The model under review builds one solid part; all positions refer to its coordinate system, in mm. A direction names the side the tool comes from. Give positions to 0.01 mm unless a question says otherwise; leave off trailing zeros. Loops run counter-clockwise (first coordinate to the right, second up) from the corner with the lowest first, then second, coordinate; pieces in that order, holes last. Notation, with made-up numbers: (81.25, 27.25) -> (110.25, 27.25) arc R33 ccw to (110.25, 57.25) -> close; hole circle Ø5 at (13.5, 23.25). An arc over 180 degrees is marked (long way). Write each question's results on one line, items separated by ' | '. Start each with the question number.
Q1. Insertion check: pin 1 Ø20.5 at (x, z) = (51.59, -68.26) entering from +Y; pin 2 Ø5 at (x, z) = (-9.5, -54.5) entering from -Y. Each pin has a flat end and moves straight along its axis. Give the tip position at first contact, or say it passes through.
Q2. We need section D-D (y = 0.65). Give the number of separate pieces and of enclosed holes in the cut face, plus the area to 3 significant figures.
Q3. Machinability: for faces 1 (the face through (-67.779, 0.391, 84.596)), 2 (the face through (-1.92, 0.39, 59.97)), which of the approach directions +Z, -Z, +X, -X, +Y, -Y give a long, thin tool a straight path to every point of the face, cutting with its end or side? Answer none if there is none.
Q4. Mouldability with a two-part tool opening along Z and no side actions: class faces 3 (the face through (48, 0.794, -21)), 4 (the face through (67.779, 0.391, -84.596)), 5 (the face through (-51.9, 0.4, 38)) as released by +Z, released by -Z, zero draft, split by the parting line, or undercut.
Q5. We need section C-C (z = -24). Write out the cut boundary in (x, y).
Q6. Wall thickness on L1, parallel to X at y = 0.6, z = 0; L2, parallel to X at y = 0.1, z = -41; L3, parallel to X at y = 0.15, z = 3.5: over which ranges is each line inside the solid? List them lowest first. Write a range as [from, to].
Q7. We need section B-B (z = 0). Write out the cut boundary in (x, y), plus the area to 3 significant figures.
Q8. We need section A-A (x = 0). Write out the cut boundary in (y, z).
from build123d import *

# Parameters (mm, degrees)
SKETCH1_R           = 12.7
SKETCH1_R_2         = 51.59375
SKETCH1_R_3         = 4.7625
SKETCH1_R_4         = 1.984375
BOSS_EXTRUDE1_DEPTH = 0.79375


with BuildPart() as part:
    # Sketch1 → Boss-Extrude1 (new body)
    with BuildSketch(Plane(origin=(0, 0, 0), x_dir=(1, 0, 0), z_dir=(0, 1, 0))):
        with BuildLine():
            Line((-61.11875, 87.3125), (61.11875, 87.3125))
            ThreePointArc((61.11875, 87.3125), (67.853942091, 84.522692091), (70.64375, 77.7875))
            Line((70.64375, 77.7875), (70.64375, -77.7875))
            ThreePointArc((70.64375, -77.7875), (67.853942091, -84.522692091), (61.11875, -87.3125))
            Line((61.11875, -87.3125), (-61.11875, -87.3125))
            ThreePointArc((-61.11875, -87.3125), (-67.853942091, -84.522692091), (-70.64375, -77.7875))
            Line((-70.64375, -77.7875), (-70.64375, 77.7875))
            ThreePointArc((-70.64375, 77.7875), (-67.853942091, 84.522692091), (-61.11875, 87.3125))
        make_face()
        with Locations(Location((-51.59375, 68.2625, 0), (0, 0, 270))):
            Circle(SKETCH1_R, mode=Mode.SUBTRACT)
        with Locations(Location((51.59375, 68.2625, 0), (0, 0, 270))):
            Circle(SKETCH1_R, mode=Mode.SUBTRACT)
        with Locations(Location((-51.59375, -68.2625, 0), (0, 0, 270))):
            Circle(SKETCH1_R, mode=Mode.SUBTRACT)
        with Locations(Location((51.59375, -68.2625, 0), (0, 0, 270))):
            Circle(SKETCH1_R, mode=Mode.SUBTRACT)
        with Locations(Location((0, 0, 0), (0, 0, 270))):
            Circle(SKETCH1_R_2, mode=Mode.SUBTRACT)
        with Locations(Location((-63.5, 0, 0), (0, 0, 270))):
            Circle(SKETCH1_R_3, mode=Mode.SUBTRACT)
        with Locations(Location((63.5, 0, 0), (0, 0, 270))):
            Circle(SKETCH1_R_3, mode=Mode.SUBTRACT)
        with Locations(Location((-63.5, -7.62, 0), (0, 0, 270))):
            Circle(SKETCH1_R_4, mode=Mode.SUBTRACT)
        with Locations(Location((63.5, -7.62, 0), (0, 0, 270))):
            Circle(SKETCH1_R_4, mode=Mode.SUBTRACT)
        with BuildLine():
            ThreePointArc((-52.47407269, 44.03097504), (-51.950230865, 38.043435583), (-45.962691407, 38.567277408))
            ThreePointArc((-45.962691407, 38.567277408), (-2.617164655, 59.942925664), (42.426429781, 42.426429781))
            ThreePointArc((42.426429781, 42.426429781), (48.436840667, 42.426429781), (48.436840667, 48.436840667))
            ThreePointArc((48.436840667, 48.436840667), (-2.987929648, 68.434840133), (-52.47407269, 44.03097504))
        make_face(mode=Mode.SUBTRACT)
        with BuildLine():
            ThreePointArc((42.426429781, -42.426429781), (-2.617164655, -59.942925664), (-45.962691407, -38.567277408))
            ThreePointArc((-45.962691407, -38.567277408), (-51.950230865, -38.043435583), (-52.47407269, -44.03097504))
            ThreePointArc((-52.47407269, -44.03097504), (-2.987929648, -68.434840133), (48.436840667, -48.436840667))
            ThreePointArc((48.436840667, -48.436840667), (48.436840667, -42.426429781), (42.426429781, -42.426429781))
        make_face(mode=Mode.SUBTRACT)
    extrude(amount=BOSS_EXTRUDE1_DEPTH)


solid = part.part
Output:
1) pin 1: through | pin 2: y = 0
2) separate pieces: 1 | enclosed holes: 11 | area: 12,100 mm2
3) face 1: +Z, -X, +Y, -Y | face 2: +Y, -Y
4) face 3: zero draft | face 4: released by -Z | face 5: undercut
5) outline: (-70.64, 0) -> (-45.67, 0) -> (-45.67, 0.79) -> (-70.64, 0.79) -> close; (45.67, 0) -> (70.64, 0) -> (70.64, 0.79) -> (45.67, 0.79) -> close
6) L1: [-70.64, -68.26], [-58.74, -51.59], [51.59, 58.74], [68.26, 70.64] | L2: [-70.64, -53.46], [-43.81, -31.32], [31.32, 70.64] | L3: [-70.64, -66.73], [-60.27, -51.47], [51.47, 60.27], [66.73, 70.64]
7) outline: (-70.64, 0) -> (-68.26, 0) -> (-68.26, 0.79) -> (-70.64, 0.79) -> close; (-58.74, 0) -> (-51.59, 0) -> (-51.59, 0.79) -> (-58.74, 0.79) -> close; (51.59, 0) -> (58.74, 0) -> (58.74, 0.79) -> (51.59, 0.79) -> close; (68.26, 0) -> (70.64, 0) -> (70.64, 0.79) -> (68.26, 0.79) -> close | area: 15.1 mm2
8) outline: (0, -87.31) -> (0.79, -87.31) -> (0.79, -68.5) -> (0, -68.5) -> close; (0, -60) -> (0.79, -60) -> (0.79, -51.59) -> (0, -51.59) -> close; (0, 51.59) -> (0.79, 51.59) -> (0.79, 60) -> (0, 60) -> close; (0, 68.5) -> (0.79, 68.5) -> (0.79, 87.31) -> (0, 87.31) -> close
